Part model, mm, in its own coordinate system. Round coordinates to 2 decimals unless told otherwise and drop trailing zeros. Order: outer loops, then holes, each group sorted by start corner. A loop starts at its lowest first (then second) coordinate and runs counter-clockwise, first axis right, second up. Notation, with made-up numbers: M -36.75,38.5 L 17.25,38.5 A21 ccw 17.25,65.5 Z; hole C 9,41.5 d11. An arc over 180 degrees is marked long. Write each question's results on one line, items separated by ' | '. Start each with the question number.
1. Band-saw the part on C-C, the plane y = 1.2. Give the number of separate pieces and of enclosed holes in the cut face, then the cut area to 3 significant figures.
2. Probe L1, parallel to X at y = 3.25, z = 52.65; L2, parallel to X at y = 1.75, z = 63; L3, parallel to X at y = 3.1, z = 2.5. List the from-to ranges inside material, lowest first. Write a range as [from, to].
3. Band-saw the part on B-B, the plane z = -63. List the corners of the cut face in (x, y), then the cut area to 3 significant figures.
4. Drop flat-ended pins along their axis: pin 1 Ø1.5 at (y, z) = (2.5, -9) entering from +X; pin 2 Ø2 at (y, z) = (1, -36.5) entering from -X. Give the stop position or say it passes through.
5. Band-saw the part on A-A, the plane x = -50. List the corners of the cut face in (y, z).
6. Band-saw the part on D-D, the plane z = 9.5. List the corners of the cut face in (x, y), then the cut area to 3 significant figures.
```python
from build123d import *

# Parameters (mm, degrees)
SKETCH1_W           = 120
SKETCH1_H           = 140
BOSS_EXTRUDE1_DEPTH = 4
SKETCH2_W           = 12
SKETCH2_H           = 23
SKETCH2_H_2         = 34
SKETCH2_R           = 1.1
SKETCH2_R_2         = 2.5
CUT_EXTRUDE1_DEPTH  = 93.28217596


with BuildPart() as part:
    # Sketch1 → Boss-Extrude1 (new body)
    with BuildSketch(Plane(origin=(0, 0, 0), x_dir=(1, 0, 0), z_dir=(0, 1, 0))):
        Rectangle(SKETCH1_W, SKETCH1_H)
    extrude(amount=BOSS_EXTRUDE1_DEPTH)

    # Sketch2 → Cut-Extrude1 (cut, through all)
    with BuildSketch(Plane(origin=(0, 4, 0), x_dir=(1, 0, 0), z_dir=(0, 1, 0))):
        with Locations((54, 38.5)):
            Rectangle(SKETCH2_W, SKETCH2_H)
        with Locations((-54, 38.5)):
            Rectangle(SKETCH2_W, SKETCH2_H)
        with Locations((54, -38.5)):
            Rectangle(SKETCH2_W, SKETCH2_H)
        with Locations((-54, -38.5)):
            Rectangle(SKETCH2_W, SKETCH2_H)
        with Locations((-54, 0)):
            Rectangle(SKETCH2_W, SKETCH2_H_2)
        with Locations((54, 0)):
            Rectangle(SKETCH2_W, SKETCH2_H_2)
        with Locations(Location((-54, 52.65, 0), (0, 0, 270))):
            Circle(SKETCH2_R)
        with Locations(Location((-54, 24.35, 0), (0, 0, 270))):
            Circle(SKETCH2_R)
        with Locations(Location((-54, -24.35, 0), (0, 0, 270))):
            Circle(SKETCH2_R)
        with Locations(Location((-54, -52.65, 0), (0, 0, 270))):
            Circle(SKETCH2_R)
        with Locations(Location((54, 52.65, 0), (0, 0, 270))):
            Circle(SKETCH2_R)
        with Locations(Location((54, 24.35, 0), (0, 0, 270))):
            Circle(SKETCH2_R)
        with Locations(Location((54, -24.35, 0), (0, 0, 270))):
            Circle(SKETCH2_R)
        with Locations(Location((54, -52.65, 0), (0, 0, 270))):
            Circle(SKETCH2_R)
        with Locations(Location((-50, 63, 0), (0, 0, 270))):
            Circle(SKETCH2_R_2)
        with Locations(Location((50, 63, 0), (0, 0, 270))):
            Circle(SKETCH2_R_2)
        with Locations(Location((50, -63, 0), (0, 0, 270))):
            Circle(SKETCH2_R_2)
        with Locations(Location((-50, -63, 0), (0, 0, 270))):
            Circle(SKETCH2_R_2)
    extrude(amount=-CUT_EXTRUDE1_DEPTH, mode=Mode.SUBTRACT)


solid = part.part
```
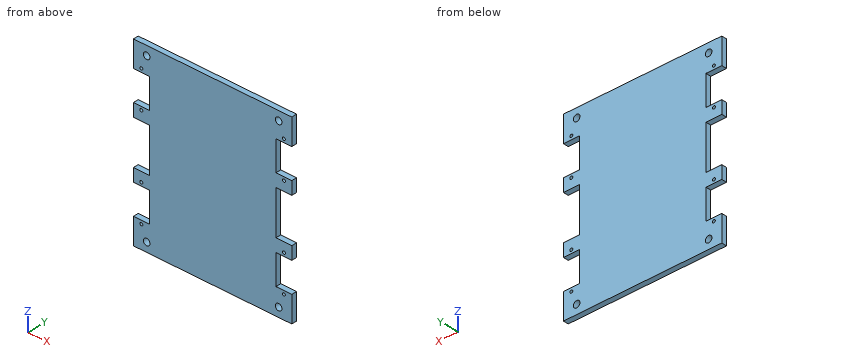
Solution:
1) separate pieces: 1 | enclosed holes: 12 | area: 14,800 mm^2
2) L1: [-60, -55.1], [-52.9, 52.9], [55.1, 60] | L2: [-60, -52.5], [-47.5, 47.5], [52.5, 60] | L3: [-48, 48]
3) outline: M -60,0 L -52.5,0 L -52.5,4 L -60,4 Z; M -47.5,0 L 47.5,0 L 47.5,4 L -47.5,4 Z; M 52.5,0 L 60,0 L 60,4 L 52.5,4 Z | area: 440 mm^2
4) pin 1: x = 48 | pin 2: x = -48
5) outline: M 0,-70 L 4,-70 L 4,-65.5 L 0,-65.5 Z; M 0,-60.5 L 4,-60.5 L 4,-50 L 0,-50 Z; M 0,-27 L 4,-27 L 4,-17 L 0,-17 Z; M 0,17 L 4,17 L 4,27 L 0,27 Z; M 0,50 L 4,50 L 4,60.5 L 0,60.5 Z; M 0,65.5 L 4,65.5 L 4,70 L 0,70 Z
6) outline: M -48,0 L 48,0 L 48,4 L -48,4 Z | area: 384 mm^2
